from build123d import *

# Parameters (mm, degrees)
EXTRUDE_3_DEPTH          = 25
SKETCH_1_5_R             = 1.65
SKETCH_1_5_R_2           = 27.5
EXTRUDE_4_DEPTH          = 3.5
CUT_EXTRUDE_1_DEPTH      = 116
CUT_EXTRUDE_1_DEPTH_BACK = 90
SKETCH_3_R               = 40.2
CUT_EXTRUDE_2_DEPTH      = 90
FILLET_1_R               = 5


with BuildPart() as part:
    # 草图1 → 凸台-拉伸3 (new body)
    with BuildSketch(Plane.XY):
        with BuildLine():
            Line((56.884812739, -66), (60, -66))
            Line((60, -66), (38.520958758, 10.776629174))
            ThreePointArc((38.520958758, 10.776629174), (0, 40), (-38.520958758, 10.776629174))
            Line((-38.520958758, 10.776629174), (-60, -66))
            Line((-60, -66), (-56.884812739, -66))
            Line((-56.884812739, -66), (-38.56602674, -0.519673214))
            ThreePointArc((-38.56602674, -0.519673214), (-38.588989549, 0.444535953), (-38.069024769, 1.256855618))
            Line((-38.069024769, 1.256855618), (-35.631886851, 9.968381986))
            ThreePointArc((-35.631886851, 9.968381986), (-32.349305917, 17.958908839), (-27.303372186, 24.970499941))
            ThreePointArc((-27.303372186, 24.970499941), (-27.329677093, 27.329677093), (-24.970499941, 27.303372186))
            ThreePointArc((-24.970499941, 27.303372186), (-14.159286998, 34.183542703), (-1.649589784, 36.963209459))
            ThreePointArc((-1.649589784, 36.963209459), (-0.018396414, 38.649897443), (1.65, 37))
            ThreePointArc((1.65, 37), (1.649897443, 36.981603586), (1.649589784, 36.963209459))
            ThreePointArc((1.649589784, 36.963209459), (14.159286998, 34.183542703), (24.970499941, 27.303372186))
            ThreePointArc((24.970499941, 27.303372186), (26.77734325, 27.694297385), (27.812950904, 26.162950904))
            ThreePointArc((27.812950904, 26.162950904), (27.680217379, 25.514566417), (27.303372186, 24.970499941))
            ThreePointArc((27.303372186, 24.970499941), (32.349305917, 17.958908839), (35.631886851, 9.968381986))
            Line((35.631886851, 9.968381986), (38.069024769, 1.256855618))
            ThreePointArc((38.069024769, 1.256855618), (38.497730094, 0.692318255), (38.65, 0))
            ThreePointArc((38.65, 0), (38.628871407, -0.263207028), (38.56602674, -0.519673214))
            Line((38.56602674, -0.519673214), (56.884812739, -66))
        make_face()
        Polygon((-60, -70), (-60, -66), (60, -66), (60, -70), (0, -70), align=None)
    extrude(amount=EXTRUDE_3_DEPTH)

    # 草图1<5> → 凸台-拉伸4 (add)
    with BuildSketch(Plane.XY):
        with BuildLine():
            Line((-56.884812739, -66), (56.884812739, -66))
            Line((56.884812739, -66), (38.56602674, -0.519673214))
            ThreePointArc((38.56602674, -0.519673214), (35.411010451, -0.444535953), (38.069024769, 1.256855618))
            Line((38.069024769, 1.256855618), (35.631886851, 9.968381986))
            ThreePointArc((35.631886851, 9.968381986), (32.349305917, 17.958908839), (27.303372186, 24.970499941))
            ThreePointArc((27.303372186, 24.970499941), (24.996224715, 24.996224715), (24.970499941, 27.303372186))
            ThreePointArc((24.970499941, 27.303372186), (14.159286998, 34.183542703), (1.649589784, 36.963209459))
            ThreePointArc((1.649589784, 36.963209459), (0, 35.35), (-1.649589784, 36.963209459))
            ThreePointArc((-1.649589784, 36.963209459), (-14.159286998, 34.183542703), (-24.970499941, 27.303372186))
            ThreePointArc((-24.970499941, 27.303372186), (-24.631604423, 26.77734325), (-24.512950904, 26.162950904))
            ThreePointArc((-24.512950904, 26.162950904), (-25.514566417, 24.645684428), (-27.303372186, 24.970499941))
            ThreePointArc((-27.303372186, 24.970499941), (-32.349305917, 17.958908839), (-35.631886851, 9.968381986))
            Line((-35.631886851, 9.968381986), (-38.069024769, 1.256855618))
            ThreePointArc((-38.069024769, 1.256855618), (-36.307681745, 1.497730094), (-35.35, 0))
            ThreePointArc((-35.35, 0), (-36.736792972, -1.628871407), (-38.56602674, -0.519673214))
            Line((-38.56602674, -0.519673214), (-56.884812739, -66))
        make_face()
        with Locations((0, -37)):
            Circle(SKETCH_1_5_R, mode=Mode.SUBTRACT)
        with Locations((-26.162950904, -26.162950904)):
            Circle(SKETCH_1_5_R, mode=Mode.SUBTRACT)
        with Locations((26.162950904, -26.162950904)):
            Circle(SKETCH_1_5_R, mode=Mode.SUBTRACT)
        Circle(SKETCH_1_5_R_2, mode=Mode.SUBTRACT)
    extrude(amount=EXTRUDE_4_DEPTH)

    # 草图2 → 切除-拉伸1 (cut, two sides: drawn at the far end of the back side and taken through both)
    with BuildSketch(Plane(origin=(0, 0, 0), x_dir=(0, 0, -1), z_dir=(1, 0, 0)).offset(-CUT_EXTRUDE_1_DEPTH_BACK)):
        Polygon((-25, -66), (-3.5, 10.776629174), (-3.5, 62.872025622), (-39.293867153, 54.574713181), (-52.271714816, -41.589010491), align=None)
    extrude(amount=CUT_EXTRUDE_1_DEPTH + CUT_EXTRUDE_1_DEPTH_BACK, mode=Mode.SUBTRACT)

    # 草图3 → 切除-拉伸2 (cut)
    with BuildSketch(Plane.XY.offset(3.5)):
        Circle(SKETCH_3_R)
    extrude(amount=CUT_EXTRUDE_2_DEPTH, mode=Mode.SUBTRACT)

    # 圆角1
    # the kernel refuses this fillet: 5 mm, written as the material it adds along each edge
    with BuildSketch(Plane(origin=(-50.294033224, -61, 8.5), x_dir=(0, -1, 0), z_dir=(0, 0, -1))) as fillet_1_piece_1_section:
        Polygon((0, 0), (FILLET_1_R, 0), (FILLET_1_R, FILLET_1_R * 1.31815590294), (-FILLET_1_R * 0.269415729351, FILLET_1_R * 0.963023968953), align=None)
    fillet_1_piece_1 = extrude(amount=FILLET_1_R, mode=Mode.PRIVATE)
    fillet_1_piece_1 = fillet_1_piece_1 - Plane(origin=(-50.294033224, -61, 8.5), x_dir=(0.7966855494331734, 0.6043940232367977, 0), z_dir=(0, 0, -1)) * Sphere(FILLET_1_R, mode=Mode.PRIVATE)
    add(fillet_1_piece_1)
    with BuildSketch(Plane(origin=(50.294033224, -61, 8.5), x_dir=(0.9630239689530686, 0.26941572935127434, 0), z_dir=(0, 0, -1))) as fillet_1_piece_2_section:
        Polygon((0, 0), (FILLET_1_R, 0), (FILLET_1_R, FILLET_1_R * 1.31815590294), (-FILLET_1_R * 0.269415729351, FILLET_1_R * 0.963023968953), align=None)
    fillet_1_piece_2 = extrude(amount=FILLET_1_R, mode=Mode.PRIVATE)
    fillet_1_piece_2 = fillet_1_piece_2 - Plane(origin=(50.294033224, -61, 8.5), x_dir=(-0.7966855494331732, 0.6043940232367977, 0), z_dir=(0, 0, -1)) * Sphere(FILLET_1_R, mode=Mode.PRIVATE)
    add(fillet_1_piece_2)
    with BuildSketch(Plane(origin=(-56.884812739, -66, 8.5), x_dir=(1, 0, 0), z_dir=(0, 0, 1))) as fillet_1_piece_3_section:
        with BuildLine():
            CenterArc((FILLET_1_R * 1.31815590294, FILLET_1_R), FILLET_1_R, 164.370497689, 105.629502311)
            Line((FILLET_1_R * 0.35513193399, FILLET_1_R * 1.26941572935), (0, 0))
            Line((0, 0), (FILLET_1_R * 1.31815590294, 0))
        make_face()
    fillet_1_piece_3 = extrude(amount=16.5, mode=Mode.PRIVATE)
    fillet_1_piece_3 = split(fillet_1_piece_3, bisect_by=Plane(origin=(-54.909873659, -62.45182584, 24.006393674), z_dir=(0, -0.26965951135538185, -0.9629557351901368)), keep=Keep.TOP, mode=Mode.PRIVATE)
    add(fillet_1_piece_3)
    with BuildSketch(Plane(origin=(56.884812739, -66, 8.5), x_dir=(-0.26941572935127367, 0.963023968953069, 0), z_dir=(0, 0, 1))) as fillet_1_piece_4_section:
        with BuildLine():
            CenterArc((FILLET_1_R * 1.31815590294, FILLET_1_R), FILLET_1_R, 164.370497689, 105.629502311)
            Line((FILLET_1_R * 0.35513193399, FILLET_1_R * 1.26941572935), (0, 0))
            Line((0, 0), (FILLET_1_R * 1.31815590294, 0))
        make_face()
    fillet_1_piece_4 = extrude(amount=16.5, mode=Mode.PRIVATE)
    fillet_1_piece_4 = split(fillet_1_piece_4, bisect_by=Plane(origin=(54.909873659, -62.45182584, 24.006393674), z_dir=(0, -0.26965951135538185, -0.9629557351901368)), keep=Keep.TOP, mode=Mode.PRIVATE)
    add(fillet_1_piece_4)
    with BuildSketch(Plane(origin=(-50.294033224, -66, 3.5), x_dir=(0, 1, 0), z_dir=(1, 0, 0))) as fillet_1_piece_5:
        with BuildLine():
            CenterArc((FILLET_1_R, FILLET_1_R), FILLET_1_R, 180, 90)
            Line((0, FILLET_1_R), (0, 0))
            Line((0, 0), (FILLET_1_R, 0))
        make_face()
    extrude(amount=100.588066449)
    with BuildSketch(Plane(origin=(-36.498733621, 6.86984643, 3.5), x_dir=(0.9630239689530686, -0.26941572935127456, 0), z_dir=(-0.26941572935127456, -0.9630239689530686, 0))) as fillet_1_piece_6_section:
        with BuildLine():
            CenterArc((FILLET_1_R, FILLET_1_R), FILLET_1_R, 180, 90)
            Line((0, FILLET_1_R), (0, 0))
            Line((0, 0), (FILLET_1_R, 0))
        make_face()
    fillet_1_piece_6 = extrude(amount=69.076959586, mode=Mode.PRIVATE)
    fillet_1_piece_6 = fillet_1_piece_6 - Plane(origin=(0, 0, 4.655624457), x_dir=(1, 0, 0), z_dir=(0, 0, -1)) * Cylinder(40.2, 159, mode=Mode.PRIVATE)
    fillet_1_piece_6 = split(fillet_1_piece_6, bisect_by=Plane(origin=(-46.735846126, -30.837467909, 15.153325978), z_dir=(0, -0.26965951135538185, -0.9629557351901368)), keep=Keep.TOP, mode=Mode.PRIVATE)
    add(fillet_1_piece_6)
    with BuildSketch(Plane(origin=(55.109153069, -59.652921353, 3.5), x_dir=(-0.9630239689530686, -0.2694157293512744, 0), z_dir=(-0.26941572935127434, 0.9630239689530686, 0))) as fillet_1_piece_7_section:
        with BuildLine():
            CenterArc((FILLET_1_R, FILLET_1_R), FILLET_1_R, 180, 90)
            Line((0, FILLET_1_R), (0, 0))
            Line((0, 0), (FILLET_1_R, 0))
        make_face()
    fillet_1_piece_7 = extrude(amount=69.076959586, mode=Mode.PRIVATE)
    fillet_1_piece_7 = fillet_1_piece_7 - Plane(origin=(0, 0, 4.655620612), x_dir=(1, 0, 0), z_dir=(0, 0, -1)) * Cylinder(40.2, 159, mode=Mode.PRIVATE)
    fillet_1_piece_7 = split(fillet_1_piece_7, bisect_by=Plane(origin=(46.735848084, -30.837472193, 15.153327178), z_dir=(0, -0.26965951135538185, -0.9629557351901368)), keep=Keep.TOP, mode=Mode.PRIVATE)
    add(fillet_1_piece_7)


solid = part.part
The model under review builds one solid part; all positions refer to its coordinate system, in mm. A direction names the side the tool comes from. Coordinates: 2 decimals unless noted, no trailing zeros. Loops run counter-clockwise (first coordinate to the right, second up) from the corner with the lowest first, then second, coordinate; pieces in that order, holes last.
(1) Consider section A-A, the plane x = 0. Give the boundary of the cut face in (y, z), plus the area to 3 significant figures.
Determined:
outline: (-70, 0) - (-38.65, 0) - (-38.65, 3.5) - (-61, 3.5) arc R5 cw to (-66, 8.5) - (-66, 25) - (-70, 25) - close; (-35.35, 0) - (-27.5, 0) - (-27.5, 3.5) - (-35.35, 3.5) - close; (27.5, 0) - (35.35, 0) - (35.35, 3.5) - (27.5, 3.5) - close; (38.65, 0) - (40, 0) - (40, 3.5) - (38.65, 3.5) - close
area: 261 mm2
(2) Consider section B-B, the plane x = 20.5. Give the boundary of the cut face in (y, z).
Determined:
outline: (-70, 0) - (-18.33, 0) - (-18.33, 3.5) - (-61, 3.5) arc R5 cw to (-66, 8.5) - (-66, 25) - (-70, 25) - close; (18.33, 0) - (34.35, 0) - (34.35, 3.5) - (18.33, 3.5) - close
(3) Draft analysis for pull direction X (two halves, no side actions). For faces 1 (the flat face through (-49.5, -39.6, 14.1)), 2 (the cylindrical face through (0.727, 39.993, 1.726)), 3 (the flat face through (48.997, -34.771, 16.255)), state which applies: +X half, -X half, draft (parallel to the pull), parting line (faces both ways), or undercut.
Determined:
face 1: undercut
face 2: parting line
face 3: draft
(4) Wall thickness on L1, parallel to X at y = 0, z = 2.3; L2, parallel to Y at x = 21, z = 22.5; L3, parallel to Z at x = -30.5, y = -16.5: over which ranges is each line inside the solid? List them lowest first.
Determined:
L1: x = -41.54 to -38.65, -35.35 to -27.5, 27.5 to 35.35, 38.65 to 41.54
L2: y = -70 to -66
L3: z = 0 to 3.5
(5) Insertion check: P1, Ø5.5, axis at x = 37, y = 0, coming from the +Z side; P2, Ø2, axis at x = 1, y = -50.5, coming from the -Z side; P3, Ø1, axis at x = 30, z = 7.5, coming from the +Y side; P4, Ø10, axis at x = 1.5, z = 18, coming from the +Y side. Each pin has a flat end and moves straight along its axis. Give the tip position at first contact, or say it passes through.
Determined:
P1: stops at z = 3.5
P2: stops at z = 0
P3: stops at y = -65.77
P4: stops at y = -66
(6) Consider section D-D, the plane x = -31. Give the boundary of the cut face in (y, z), plus the area to 3 significant figures.
Determined:
outline: (-70, 0) - (25.28, 0) - (25.28, 3.5) - (-61, 3.5) arc R5 cw to (-66, 8.5) - (-66, 25) - (-70, 25) - close
area: 425 mm2
(7) Tool access review of faces 4 (the cylindrical face through (-46, -32.4, 5)), 5 (the cylindrical face through (0.89, -35.61, 1.73)): name each direction out of +Z, -Z, +X, -X, +Y, -Y from which nothing blocks a thin tool from reaching the whole face with its end or side.
Determined:
face 4: +Z
face 5: +Z, -Z
(8) Consider section C-C, the plane z = 19.75. Give the boundary of the cut face in (x, y), plus the area to 3 significant figures.
Determined:
outline: (-60, -70) - (60, -70) - (60, -66) - (54.76, -47.25) - (51.64, -47.25) - (55.11, -59.65) arc R5 cw to (50.29, -66) - (-50.29, -66) arc R5 cw to (-55.11, -59.65) - (-51.64, -47.25) - (-54.76, -47.25) - (-60, -66) - close
area: 617 mm2
